Can you work these out from the model? Positions are in its coordinate system, mm. A direction names the side the tool comes from. Round coordinates to 2 decimals unless told otherwise and drop trailing zeros. Write each loop counter-clockwise with the first axis right and the second up, starting at its lowest first coordinate (ties: lowest second). Pieces come first, ordered by that corner, then holes.
Q1. If we section it at B-B (y = 0): Please give me the cut outline in (x, z).
Q2. For faces 5 (the flat face through (57.451, 0, 20)), 6 (the cylindrical face through (-0.559, -35.427, 15.603)), 7 (the cylindrical face through (0.559, 35.427, 15.603)), which set-ups out of +Z, -Z, +X, -X, +Y, -Y let a thin tool reach every point of the face, with its end or its side?
Q3. I'm going to push a flat-ended pin straight in: pin 1 Ø20.5 at (x, z) = (8, 10.5) entering from -Y. Where does the tip first touch, or does it pass through?
Q4. If we section it at C-C (z = 11.5): Please give me the cut outline in (x, y), plus the area to 3 significant figures.
Q5. If we section it at A-A (z = 37.5): Please give me the cut outline in (x, y).
Q6. Please list where these lines run through material, in increasing order: line 1 along Y through (x, z) = (30, 10.5); line 2 along X through (y, z) = (3.5, 8); line 3 along X through (y, z) = (-6.5, 34).
Q7. We'd pull the mould along Y, two halves only. Please class faces 1 (the flat face through (-1, 30.497, 11)), 2 (the cylindrical face through (35.24, 0.32, 20.21)), 3 (the flat face through (0, -40.497, 23)), 4 (the flat face through (-57.451, 0, 20)): +Y half, -Y half, draft (parallel to the pull), parting line (faces both ways), or undercut.
Q8. If we section it at D-D (x = 0): Please give me the cut outline in (y, z).
from build123d import *

# Parameters (mm, degrees)
F0_W     = 114.9016693234
F0_H     = 60.9933659434
F0_R     = 7.2773079639
F1_DEPTH = 41
F3_DEPTH = 60.9943659434
F4_DEPTH = 10
F6_DEPTH = 10


with BuildPart() as f1:
    # F0 (on Top) → F1 (new body)
    with BuildSketch(Plane.XY):
        Rectangle(F0_W, F0_H)
        with Locations((-42.510535568, 0)):
            Circle(F0_R, mode=Mode.SUBTRACT)
        with Locations((42.510535568, 0)):
            Circle(F0_R, mode=Mode.SUBTRACT)
    extrude(amount=F1_DEPTH)

    # F2 (on face) → F3 (cut, through all)
    with BuildSketch(Plane.XZ.offset(30.4966829717)):
        with BuildLine():
            ThreePointArc((-17.4030642732, 41), (0, 23.5969357268), (17.4030642732, 41))
            Line((17.4030642732, 41), (-17.4030642732, 41))
        make_face()
    extrude(amount=-F3_DEPTH, mode=Mode.SUBTRACT)

    # F2 (on face) → F4 (join)
    with BuildSketch(Plane.XZ.offset(30.4966829717)):
        with BuildLine():
            Line((25.4030636924, 41), (17.4030642732, 41))
            ThreePointArc((17.4030642732, 41), (0, 23.5969357268), (-17.4030642732, 41))
            Line((-17.4030642732, 41), (-25.4030636924, 41))
            ThreePointArc((-25.4030636924, 41), (0, 15.5969363076), (25.4030636924, 41))
        make_face()
    extrude(amount=F4_DEPTH)

    # F5 (on face) → F6 (join)
    with BuildSketch(Plane(origin=(0, 30.4966829717, 0), x_dir=(-1, 0, 0), z_dir=(0, 1, 0))):
        with BuildLine():
            ThreePointArc((-25.4030636924, 41), (0, 15.5969363076), (25.4030636924, 41))
            Line((25.4030636924, 41), (17.4030642732, 41))
            ThreePointArc((17.4030642732, 41), (0, 23.5969357268), (-17.4030642732, 41))
            Line((-17.4030642732, 41), (-25.4030636924, 41))
        make_face()
    extrude(amount=F6_DEPTH)


solid = f1.part
A:
1. outline: (-57.45, 0) - (-49.79, 0) - (-49.79, 41) - (-57.45, 41) - close; (-35.23, 0) - (35.23, 0) - (35.23, 41) - (17.4, 41) arc R17.4 cw to (-17.4, 41) - (-35.23, 41) - close; (49.79, 0) - (57.45, 0) - (57.45, 41) - (49.79, 41) - close
2. face 5: +Z, -Z, +X, +Y, -Y
2. face 6: -Z, -Y
2. face 7: -Z, +Y
3. pin 1: stops at y = -40.5
4. outline: (-57.45, -30.5) - (57.45, -30.5) - (57.45, 30.5) - (-57.45, 30.5) - close; hole circle Ø14.55 at (-42.51, 0); hole circle Ø14.55 at (42.51, 0)
4. area: 6,680 mm2
5. outline: (-57.45, -30.5) - (-25.16, -30.5) - (-25.16, -40.5) - (-17.05, -40.5) - (-17.05, 40.5) - (-25.16, 40.5) - (-25.16, 30.5) - (-57.45, 30.5) - close; (17.05, -40.5) - (25.16, -40.5) - (25.16, -30.5) - (57.45, -30.5) - (57.45, 30.5) - (25.16, 30.5) - (25.16, 40.5) - (17.05, 40.5) - close; hole circle Ø14.55 at (-42.51, 0); hole circle Ø14.55 at (42.51, 0)
6. line 1: y = -30.5 to 30.5
6. line 2: x = -57.45 to -48.89, -36.13 to 36.13, 48.89 to 57.45
6. line 3: x = -57.45 to -45.78, -39.24 to -15.93, 15.93 to 39.24, 45.78 to 57.45
7. face 1: +Y half
7. face 2: undercut
7. face 3: -Y half
7. face 4: draft
8. outline: (-40.5, 15.6) - (-30.5, 15.6) - (-30.5, 0) - (30.5, 0) - (30.5, 15.6) - (40.5, 15.6) - (40.5, 23.6) - (-40.5, 23.6) - close
